Source: CAD feature listing. Evaluate the final solid. Frame: model axes, mm. A direction names the side the tool comes from. Coordinates: 2 decimals unless noted, no trailing zeros. Write each loop counter-clockwise with the first axis right and the second up, starting at its lowest first coordinate (ties: lowest second). Pieces come first, ordered by that corner, then holes. Notation, with made-up numbers: (-20.75, -17.75) - (10.25, -17.75) arc R21 cw to (10.25, -2.75) - close; hole circle Ø9 at (4.5, -9.75). An arc over 180 degrees is marked (long way). One line per item, written item: value.
from build123d import *

# Parameters (mm, degrees)
ESQUISSE1_W        = 400
ESQUISSE1_H        = 400
ESQUISSE1_R        = 150
BOSS_EXTRU_1_DEPTH = 5
BOSS_EXTRU_2_START = -5
BOSS_EXTRU_2_DEPTH = 5
BOSS_EXTRU_3_DEPTH = 5


with BuildPart() as part:
    # Esquisse1 → Boss.-Extru.1 (new body)
    with BuildSketch(Plane(origin=(0, 0, 0), x_dir=(0, 0, -1), z_dir=(1, 0, 0))):
        Rectangle(ESQUISSE1_W, ESQUISSE1_H)
        Circle(ESQUISSE1_R, mode=Mode.SUBTRACT)
    extrude(amount=BOSS_EXTRU_1_DEPTH)

    # Esquisse2 → Boss.-Extru.2 (add)
    with BuildSketch(Plane(origin=(5, 0, 0), x_dir=(0, 0, -1), z_dir=(1, 0, 0)).offset(BOSS_EXTRU_2_START)):
        with BuildLine():
            ThreePointArc((-149.963113542, 3.326345848), (-83.411685222, 60.117854594), (-50.582353171, 141.214112424))
            ThreePointArc((-50.582353171, 141.214112424), (-121.687633298, 87.704731357), (-149.963113542, 3.326345848))
        make_face()
    extrude(amount=BOSS_EXTRU_2_DEPTH)

    # Esquisse3 → Boss.-Extru.3 (add)
    with BuildSketch(Plane(origin=(5, 0, 0), x_dir=(0, 0, -1), z_dir=(1, 0, 0))):
        with BuildLine():
            Line((-50.641756069, 68.696951836), (-49.121294777, 64.950100794))
            add(Edge.make_bspline(
                [(-49.121294777, 64.950100794), (-52.51075488, 63.09305926), (-56.251037239, 54.874213626), (-55.436032913, 45.973549374), (-53.544421741, 41.460575016)],
                knots=[0, 0, 0, 0, 0.427817388, 1, 1, 1, 1], degree=3))
            add(Edge.make_bspline(
                [(-53.544421741, 41.460575016), (-49.493771524, 43.143934267), (-43.677837846, 47.551694172), (-40.650983319, 57.726456605), (-43.687514554, 64.208576547), (-47.151888648, 65.394746752)],
                knots=[0, 0, 0, 0, 0.433456204, 0.652391978, 1, 1, 1, 1], degree=3))
            Line((-47.151888648, 65.394746752), (-47.473938049, 67.920044269))
            Line((-47.473938049, 67.920044269), (-29.771089937, 63.143994688))
            Line((-29.771089937, 63.143994688), (-27.162840794, 59.083409632))
            Line((-27.162840794, 59.083409632), (-26.639406106, 62.322569421))
            Line((-26.639406106, 62.322569421), (-22.121567137, 60.423023491))
            add(Edge.make_bspline(
                [(-22.121567137, 60.423023491), (-21.900652986, 58.844405298), (-22.593906313, 56.188877616), (-20.433988328, 53.424341294), (-19.157824546, 49.900753611), (-18.893704947, 46.014732552), (-16.715964955, 43.373118799), (-16.761241643, 40.99576311), (-14.932536534, 39.250943841), (-13.221453122, 35.220671727), (-8.354015779, 34.949952489), (-6.866737858, 37.536191267)],
                knots=[0, 0, 0, 0, 0.150869305, 0.214819056, 0.309773428, 0.491679736, 0.556111964, 0.609109072, 0.695847406, 0.772434776, 1, 1, 1, 1], degree=3))
            Line((-6.866737858, 37.536191267), (-5.513363019, 35.834805755))
            Line((-5.513363019, 35.834805755), (-1.768809898, 38.243418268))
            Line((-1.768809898, 38.243418268), (2.613795129, 38.243418268))
            Line((2.613795129, 38.243418268), (6.468274065, 39.713813265))
            Line((6.468274065, 39.713813265), (8.184977276, 41.64986563))
            Line((8.184977276, 41.64986563), (11.445710099, 41.275068754))
            add(Edge.make_bspline(
                [(11.445710099, 41.275068754), (12.91703059, 41.729549687), (14.682145059, 45.752837691), (14.248125034, 49.630437287), (13.942831767, 52.154597518)],
                knots=[0, 0, 0, 0, 0.363892157, 1, 1, 1, 1], degree=3))
            add(Edge.make_bspline(
                [(13.942831767, 52.154597518), (15.106729387, 53.423805744), (15.81295353, 55.843879283), (16.578340557, 59.892537097), (15.323868262, 62.437984958), (13.495569111, 62.795247815)],
                knots=[0, 0, 0, 0, 0.408732991, 0.60243167, 1, 1, 1, 1], degree=3))
            add(Edge.make_bspline(
                [(13.495569111, 62.795247815), (13.970078, 63.802995831), (15.705345795, 67.184562867), (12.041497459, 70.287418684), (10.116975826, 70.632248522)],
                knots=[0, 0, 0, 0, 0.344176041, 1, 1, 1, 1], degree=3))
            Line((10.116975826, 70.632248522), (3.494410121, 70.632248522))
            add(Edge.make_bspline(
                [(3.494410121, 70.632248522), (1.786435249, 73.243810631), (0.841555231, 76.383068781), (-1.984622914, 78.154912931)],
                knots=[0, 0, 0, 0, 1, 1, 1, 1], degree=3))
            add(Edge.make_bspline(
                [(-1.984622914, 78.154912931), (-4.619654468, 76.485525149), (-9.255881643, 75.250433561), (-16.519433272, 71.568054765), (-17.480141985, 66.153041817), (-20.733248382, 65.394746752)],
                knots=[0, 0, 0, 0, 0.395717089, 0.631602506, 1, 1, 1, 1], degree=3))
            Line((-20.733248382, 65.394746752), (-36.731609625, 68.966498574))
            Line((-36.731609625, 68.966498574), (-35.254584345, 70.632248522))
            add(Edge.make_bspline(
                [(-35.254584345, 70.632248522), (-33.26309679, 70.210780339), (-28.028974684, 72.174025739), (-27.339523708, 72.730784764), (-25.299138881, 75.206231145), (-23.154125649, 79.109230145), (-22.637221031, 84.197953328), (-23.001491077, 87.035020266)],
                knots=[0, 0, 0, 0, 0.05163777, 0.199516391, 0.247017501, 0.508164038, 1, 1, 1, 1], degree=3))
            add(Edge.make_bspline(
                [(-23.001491077, 87.035020266), (-27.142409249, 87.753037067), (-32.808173774, 85.571818964), (-38.094245187, 78.91770696), (-38.086684666, 74.341614121), (-37.646065549, 71.823781121)],
                knots=[0, 0, 0, 0, 0.488970635, 0.684624182, 1, 1, 1, 1], degree=3))
            Line((-37.646065549, 71.823781121), (-39.987885316, 69.960969942))
            Line((-39.987885316, 69.960969942), (-49.705455686, 72.944960143))
            Line((-49.705455686, 72.944960143), (-47.473938049, 75.865174629))
            Line((-47.473938049, 75.865174629), (-52.728820416, 73.810875285))
            add(Edge.make_bspline(
                [(-52.728820416, 73.810875285), (-65.290226854, 77.416651114), (-74.909544365, 88.095525002), (-82.830465292, 97.70673649)],
                knots=[0, 0, 0, 0, 1, 1, 1, 1], degree=3))
            Line((-82.830465292, 97.70673649), (-88.369376858, 87.035020266))
            add(Edge.make_bspline(
                [(-88.369376858, 87.035020266), (-72.280582145, 71.618587652), (-50.641756069, 68.696951836)],
                knots=[0, 0, 0, 1, 1, 1], degree=2))
        make_face()
    extrude(amount=-BOSS_EXTRU_3_DEPTH)


solid = part.part
1) Section query B-B on y = 129. Output: boundary loops of the cut face in (x, z), then the cut area to 3 significant figures.
Values found:
outline: (0, -200) - (5, -200) - (5, -76.54) - (0, -76.54) - close; (0, 52.79) - (5, 52.79) - (5, 200) - (0, 200) - close
area: 1,350 mm2
2) Material intervals for line 1 (Z direction, x = 3.3, y = 0); line 2 (Z direction, x = 4.6, y = -126); line 3 (Y direction, x = 4.3, z = 13), sorted ascending.
Values found:
line 1: -200 to -150, 150 to 200
line 2: -200 to -81.39, 81.39 to 200
line 3: -200 to -149.44, 36.39 to 73.23, 149.44 to 200
3) Draft query along Z for faces 1 (the flat face through (0, 47, 3)), 2 (the cylindrical face through (2.465, 111.044, 57.615)). Return one class per face: released by +Z, released by -Z, zero draft, split by the parting line, or undercut.
Values found:
face 1: zero draft
face 2: undercut
4) Reachability of faces 3 (the cylindrical face through (2.5, 33.5, 106.8)), 4 (the flat face through (5, 47, 3)) from +Z, -Z, +X, -X, +Y, -Y: full face, straight path, thin tool, end or side. Return the list, or none.
Values found:
face 3: +X, -X
face 4: +Z, -Z, +X, +Y, -Y
5) Section query A-A on z = -130. Output: boundary loops of the cut face in (x, y).
Values found:
outline: (0, -200) - (5, -200) - (5, -74.83) - (0, -74.83) - close; (0, 74.83) - (5, 74.83) - (5, 200) - (0, 200) - close
